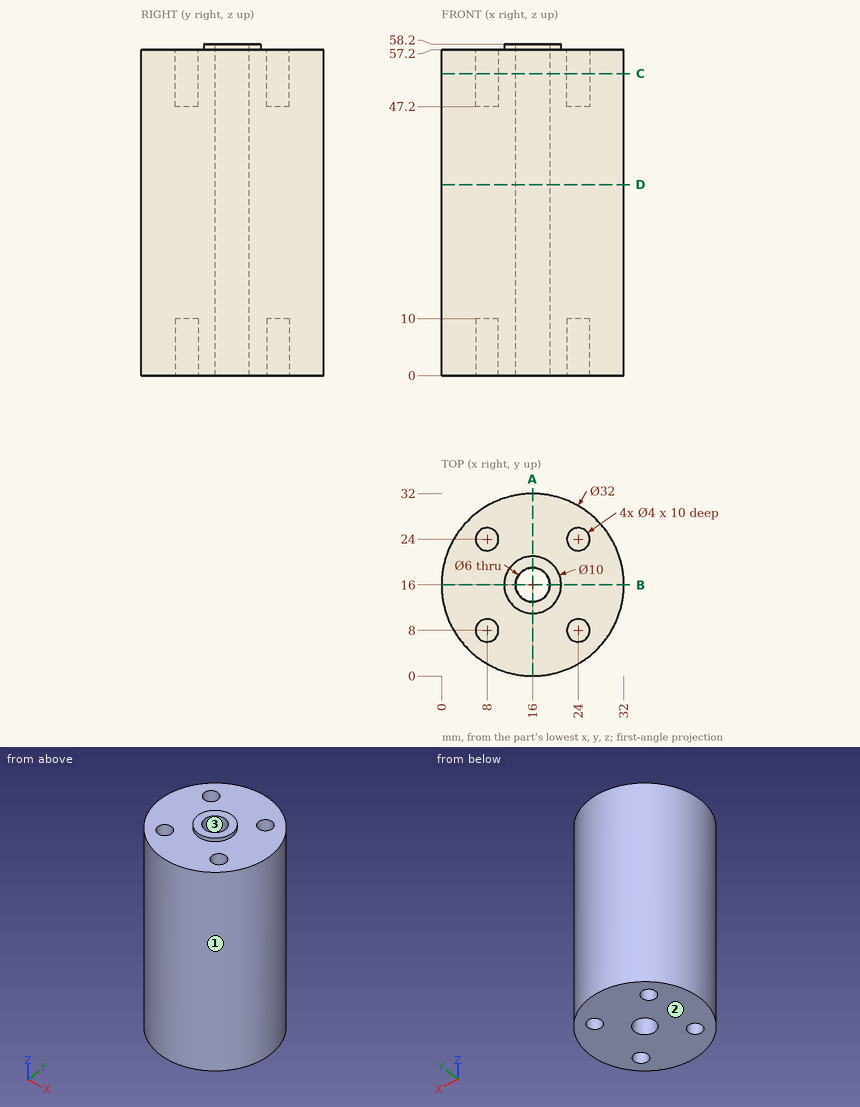
Answer from the drawing. Dimensions are ordinates in mm from the lowest x, y and z of the part. Round coordinates to 2 decimals unless told otherwise and drop trailing zeros. Write each loop counter-clockwise with the first axis right and the second up, starting at its lowest first coordinate (ties: lowest second). Pieces come first, ordered by that corner, then holes. Notation, with made-up numbers: (80.25, -4) -> (122.25, -4) arc R17 cw to (122.25, 16) -> close; hole circle Ø8 at (41, 77). An arc over 180 degrees is marked (long way). Answer in a Markdown table with one row per item. Add a question column.
1) Consider line 1 (Z direction, x = 3.5, y = 20); line 2 (Y direction, x = 18.5, z = 5.5); line 3 (Y direction, x = 15, z = 16). Determine where each line is inside the solid, lowest interval first.
2) Find section C-C, the plane z = 53. Determine the outline of the cut face in (x, y), and give its area (3 significant figures).
3) Determine the mould class of the marked faces 1, 2 and 3 for opening direction X: pulls with the +X half, pulls with the -X half, needs draft (parallel to the pull), parting line crosses it, or undercut.
4) Find section D-D, the plane z = 33.5. Determine the outline of the cut face in (x, y), and give its area (3 significant figures).
5) Find section A-A, the plane x = 16. Determine the outline of the cut face in (y, z), and give its area (3 significant figures).
6) Given P1, Ø2, axis at x = 24.5, y = 9, coming from the +Z side; P2, Ø2, axis at x = 7.5, y = 24.5, coming from the +Z side; P3, Ø4, axis at x = 10, z = 46.5, coming from the +Y side, each flat-ended and moving along its own axis, determine where each tip first touches the part or whether it passes through.
Findings below:
| question | item | result |
|---|---|---|
| 1 | line 1 | 0 to 57.2 |
| 1 | line 2 | 0.2 to 14.34, 17.66 to 31.8 |
| 1 | line 3 | 0.03 to 13.17, 18.83 to 31.97 |
| 2 | outline | circle Ø32 at (16, 16); hole circle Ø4 at (8, 8); hole circle Ø4 at (8, 24); hole circle Ø6 at (16, 16); hole circle Ø4 at (24, 8); hole circle Ø4 at (24, 24) |
| 2 | area | 726 mm² |
| 3 | face 1 | parting line crosses it |
| 3 | face 2 | needs draft |
| 3 | face 3 | undercut |
| 4 | outline | circle Ø32 at (16, 16); hole circle Ø6 at (16, 16) |
| 4 | area | 776 mm² |
| 5 | outline | (0, 0) -> (13, 0) -> (13, 58.2) -> (11, 58.2) -> (11, 57.2) -> (0, 57.2) -> close; (19, 0) -> (32, 0) -> (32, 57.2) -> (21, 57.2) -> (21, 58.2) -> (19, 58.2) -> close |
| 5 | area | 1,490 mm² |
| 6 | P1 | z = 57.2 |
| 6 | P2 | z = 47.2 |
| 6 | P3 | y = 31.49 |
